```python
from build123d import *

# Parameters (mm, degrees)
SKETCH_1_R          = 12.25
SKETCH_1_R_2        = 1.5
EXTRUDE_1_DEPTH     = 2
SKETCH_2_R          = 5
SKETCH_2_R_2        = 3
EXTRUDE_2_DEPTH     = 3
EXTRUDE_3_DEPTH     = 2
SKETCH_4_R          = 1.5
CUT_EXTRUDE_1_DEPTH = 10
CUT_EXTRUDE_START   = -10
CUT_EXTRUDE_4_DEPTH = 10


with BuildPart() as part:
    # 草图1 → 凸台-拉伸1 (new body)
    with BuildSketch(Plane.XY):
        Circle(SKETCH_1_R)
        Circle(SKETCH_1_R_2, mode=Mode.SUBTRACT)
    extrude(amount=EXTRUDE_1_DEPTH)

    # 草图2 → 凸台-拉伸2 (add)
    with BuildSketch(Plane.XY.offset(2)):
        Circle(SKETCH_2_R)
        Circle(SKETCH_2_R_2, mode=Mode.SUBTRACT)
    extrude(amount=EXTRUDE_2_DEPTH)

    # 草图3 → 凸台-拉伸3 (add)
    with BuildSketch(Plane(origin=(0, 0, 0), x_dir=(-1, 0, 0), z_dir=(0, 0, -1))):
        with BuildLine():
            Line((12.030570384, -2.308219276), (-12.030570384, -2.308219276))
            Line((-12.030570384, -2.308219276), (-4.910436892, -39.418760727))
            ThreePointArc((-4.910436892, -39.418760727), (0, -43.47663041), (4.910436892, -39.418760727))
            Line((4.910436892, -39.418760727), (12.030570384, -2.308219276))
        make_face()
    extrude(amount=-EXTRUDE_3_DEPTH)

    # 草图4 → 切除-拉伸1 (cut)
    with BuildSketch(Plane(origin=(0, 0, 0), x_dir=(-1, 0, 0), z_dir=(0, 0, -1))):
        with Locations((7, 0)):
            Circle(SKETCH_4_R)
        with Locations((0, -7)):
            Circle(SKETCH_4_R)
        with Locations((-7, 0)):
            Circle(SKETCH_4_R)
        with Locations((0, 7)):
            Circle(SKETCH_4_R)
    extrude(amount=-CUT_EXTRUDE_1_DEPTH, mode=Mode.SUBTRACT)

    # 草图6 → 切除-拉伸4 (cut)
    with BuildSketch(Plane.XY.offset(2).offset(CUT_EXTRUDE_START)):
        with BuildLine():
            ThreePointArc((12.25, 0), (0, -12.25), (-12.25, 0))
            Line((-12.25, 0), (-14.856850111, -46.424662629))
            Line((-14.856850111, -46.424662629), (15.079980512, -43.09327684))
            Line((15.079980512, -43.09327684), (12.25, 0))
        make_face()
    extrude(amount=CUT_EXTRUDE_4_DEPTH, mode=Mode.SUBTRACT)


solid = part.part
```
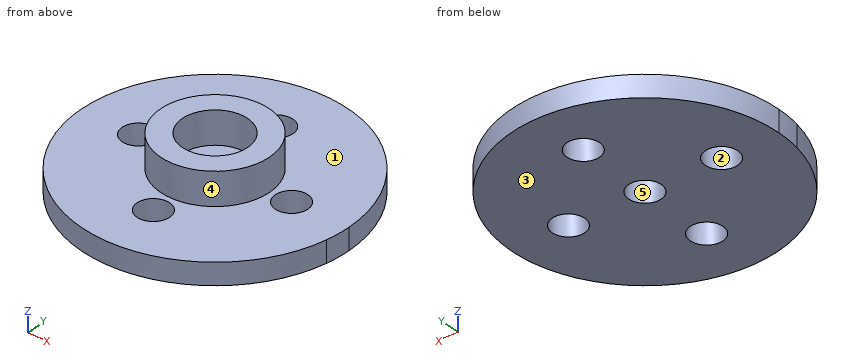
Work out the finished part from the listing and answer in its coordinate system (mm). Face numbers are marked on the shaded views. A direction names the side the tool comes from. Coordinates: 2 decimals unless noted, no trailing zeros. Loops run counter-clockwise (first coordinate to the right, second up) from the corner with the lowest first, then second, coordinate; pieces in that order, holes last. Notation, with made-up numbers: M 49.5,74 L 105.5,74 A30 cw 105.5,113 Z; hole C 29.5,64 d7. An arc over 180 degrees is marked long. Use CSV: the item, a comma, the result in double quotes. Start each with the question number.
(1) Find section A-A, the plane x = 0. Give the vertices of the cut face in (y, z), then the cut area to 3 significant figures.
(2) For the marked faces 1 and 2, determine the directions among +Z, -Z, +X, -X, +Y, -Y from which every point of the face is accessible in a straight line to the end or side of a thin tool.
(3) Consider line 1 (Y direction, x = 0, z = 1.2); line 2 (Y direction, x = 0, z = 2.75); line 3 (Z direction, x = -2.75, y = -7). Determine where each line is inside the solid, lowest interval first.
(4) Find section C-C, the plane y = 7. Give the vertices of the cut face in (x, z), then the cut area to 3 significant figures.
(5) Given pin 1 Ø3 at (x, z) = (-4.5, 1) entering from -Y; pin 2 Ø3 at (x, y) = (-1, 0) entering from +Z; pin 3 Ø2 at (x, z) = (2.5, 4) entering from -Y, each flat-ended and moving along its own axis, determine where each tip first touches the part or whether it passes through.
(6) For a pull along Y with two mould halves and no side action, classify the marked faces 3, 4 and 5 as +Y half, -Y half, draft (parallel to the pull), parting line (faces both ways), or undercut.
(7) Find section B-B, the plane z = 1.1. Give the vertices of the cut face in (x, y), then the cut area to 3 significant figures.
Recorded:
1,outline,"M -12.25,0 L -8.5,0 L -8.5,2 L -12.25,2 Z; M -5.5,0 L -1.5,0 L -1.5,2 L -3,2 L -3,5 L -5,5 L -5,2 L -5.5,2 Z; M 1.5,0 L 5.5,0 L 5.5,2 L 5,2 L 5,5 L 3,5 L 3,2 L 1.5,2 Z; M 8.5,0 L 12.25,0 L 12.25,2 L 8.5,2 Z"
1,area,"43.0 mm^2"
2,face 1,"+Z"
2,face 2,"+Z, -Z"
3,line 1,"y = -12.25 to -8.5, -5.5 to -1.5, 1.5 to 5.5, 8.5 to 12.25"
3,line 2,"y = -5 to -3, 3 to 5"
3,line 3,"z = 0 to 2"
4,outline,"M -10.05,0 L -1.5,0 L -1.5,2 L -10.05,2 Z; M 1.5,0 L 10.05,0 L 10.05,2 L 1.5,2 Z"
4,area,"34.2 mm^2"
5,pin 1,"stops at y = -11.88"
5,pin 2,"stops at z = 2"
5,pin 3,"stops at y = -4.77"
6,face 3,"draft"
6,face 4,"parting line"
6,face 5,"undercut"
7,outline,"C 0,0 d24.5; hole C -7,0 d3; hole C 0,-7 d3; hole C 0,0 d3; hole C 0,7 d3; hole C 7,0 d3"
7,area,"436 mm^2"
